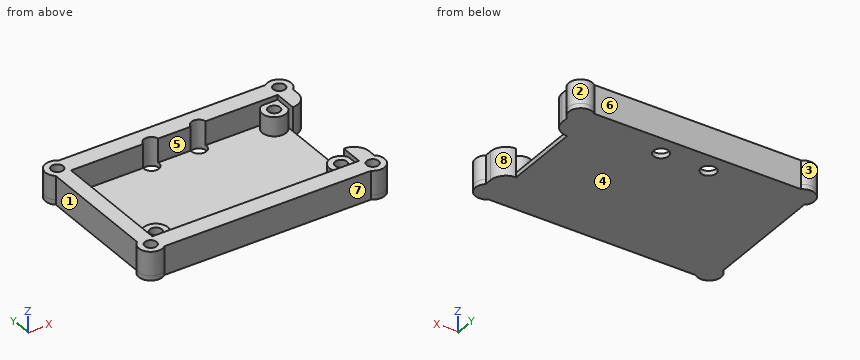
from build123d import *

# Parameters (mm, degrees)
SKETCH_R                   = 2.5
SKETCH_W                   = 87
SKETCH_H                   = 51
PAD_DEPTH                  = 10
POCKET_DEPTH               = 10.001
PAD001_DEPTH               = 2
SKETCH003_R                = 2.5
PAD002_DEPTH               = 8
SKETCH003_MIRRORED001_2_R  = 2.5
PAD002_MIRRORED001_2_DEPTH = 8
SKETCH004_R                = 3.2
POCKET001_DEPTH            = 12.001
POCKET004_DEPTH            = 8


with BuildPart() as part:
    # Sketch → Pad (new body)
    with BuildSketch(Plane.XY):
        with BuildLine():
            Line((-43.499999, 33.160444), (43.499999, 33.160444))
            ThreePointArc((49.927876, 25.500001), (50.544139, 32.544145), (43.499999, 33.160444))
            Line((49.927876, 25.500001), (49.927876, -25.500001))
            ThreePointArc((43.499999, -33.160444), (50.544159, -32.544162), (49.927876, -25.500001))
            Line((43.499999, -33.160444), (-43.499999, -33.160444))
            ThreePointArc((-49.927876, -25.500001), (-50.544159, -32.544162), (-43.499999, -33.160444))
            Line((-49.927876, -25.500001), (-49.927876, 25.500001))
            ThreePointArc((-43.499999, 33.160444), (-50.544159, 32.544162), (-49.927876, 25.500001))
        make_face()
        with Locations((-46.713937, 29.330223)):
            Circle(SKETCH_R, mode=Mode.SUBTRACT)
        with Locations((46.713917, 29.330206)):
            Circle(SKETCH_R, mode=Mode.SUBTRACT)
        with Locations((46.713937, -29.330223)):
            Circle(SKETCH_R, mode=Mode.SUBTRACT)
        with Locations((-46.713937, -29.330223)):
            Circle(SKETCH_R, mode=Mode.SUBTRACT)
        Rectangle(SKETCH_W, SKETCH_H, mode=Mode.SUBTRACT)
    extrude(amount=PAD_DEPTH)

    # Sketch001 (on Face18 of Pad) → Pocket (cut, through all)
    with BuildSketch(Plane.XY.offset(10)):
        with BuildLine():
            ThreePointArc((43.5, 16), (48.045195, 17.882681), (49.927876, 22.427876))
            Line((49.927876, 22.427876), (49.927876, -22.427876))
            ThreePointArc((49.927876, -22.427876), (48.045195, -17.882681), (43.5, -16))
            Line((43.5, 16), (43.5, -16))
        make_face()
    extrude(amount=-POCKET_DEPTH, mode=Mode.SUBTRACT)

    # Sketch002 (on Face4 of Pocket) → Pad001 (join)
    with BuildSketch(Plane(origin=(0, 0, 0), x_dir=(1, 0, 0), z_dir=(0, 0, -1))):
        with BuildLine():
            ThreePointArc((-43.499999, 33.160444), (-50.544168, 32.544169), (-49.927876, 25.500001))
            Line((-49.927876, 0), (-49.927876, 25.500001))
            Line((43.5, 0), (-49.927876, 0))
            Line((43.5, 16), (43.5, 0))
            ThreePointArc((43.5, 16), (48.045195, 17.882681), (49.927876, 22.427876))
            Line((49.927876, 25.500001), (49.927876, 22.427876))
            ThreePointArc((49.927876, 25.500001), (50.544166, 32.544167), (43.499999, 33.160444))
            Line((-43.499999, 33.160444), (43.499999, 33.160444))
        make_face()
    pad001 = extrude(amount=PAD001_DEPTH)

    # Mirrored: Pad001 across XZ
    add(pad001.mirror(Plane.XZ))

    # Sketch003 (on Face31 of Mirrored) → Pad002 (join)
    with BuildSketch(Plane.XY):
        with BuildLine():
            Line((36.820551, 25.5), (43.5, 25.5))
            Line((43.5, 25.5), (43.5, 18.820551))
            ThreePointArc((36.820551, 25.5), (35.464466, 17.464466), (43.5, 18.820551))
        make_face()
        with Locations((39, 21)):
            Circle(SKETCH003_R, mode=Mode.SUBTRACT)
    pad002 = extrude(amount=PAD002_DEPTH)

    # Sketch003 Mirrored001 2 → Pad002 Mirrored001 2 (add)
    with BuildSketch(Plane(origin=(0, 0, 0), x_dir=(-1, 0, 0), z_dir=(0, 0, -1))):
        with BuildLine():
            Line((36.820551, 25.5), (43.5, 25.5))
            Line((43.5, 25.5), (43.5, 18.820551))
            ThreePointArc((36.820551, 25.5), (35.464466, 17.464466), (43.5, 18.820551))
        make_face()
        with Locations((39, 21)):
            Circle(SKETCH003_MIRRORED001_2_R, mode=Mode.SUBTRACT)
    pad002_mirrored001_2 = extrude(amount=-PAD002_MIRRORED001_2_DEPTH)

    # Mirrored002: Pad002, Pad002 Mirrored001 2 across Sketch003 H_Axis
    add(pad002.mirror(Plane.ZX))
    add(pad002_mirrored001_2.mirror(Plane.ZX))

    # Sketch004 (on Face8 of MultiTransform) → Pocket001 (cut, through all)
    with BuildSketch(Plane(origin=(0, 0, -2), x_dir=(1, 0, 0), z_dir=(0, 0, -1))):
        with Locations((-10, -25)):
            Circle(SKETCH004_R)
        with Locations((10, -25)):
            Circle(SKETCH004_R)
    extrude(amount=-POCKET001_DEPTH, mode=Mode.SUBTRACT)

    # Sketch011 (on Face36 of Pocket001) → Pocket004 (cut)
    with BuildSketch(Plane.XY.offset(8)):
        with BuildLine():
            Line((-36.820551, 25.5), (-43.5, 25.5))
            Line((-43.5, 25.5), (-43.5, 18.820551))
            ThreePointArc((-43.5, 18.820551), (-35.464466, 17.464466), (-36.820551, 25.5))
        make_face()
    extrude(amount=-POCKET004_DEPTH, mode=Mode.SUBTRACT)


with BuildPart() as part_1:
    # Body placement: moved
    add(part.part.moved(Location((0, 0, -8))))


solid = part_1.part
The model under review builds one solid part; all positions refer to its coordinate system, in mm. Face numbers are marked on the shaded views. A direction names the side the tool comes from. Give positions to 0.01 mm unless a question says otherwise; leave off trailing zeros. Write each loop counter-clockwise with the first axis right and the second up, starting at its lowest first coordinate (ties: lowest second). Pieces come first, ordered by that corner, then holes. Notation, with made-up numbers: M -5,-1.5 L 32,-1.5 A26 cw 32,25.5 Z; hole C 66,32.5 d7. An arc over 180 degrees is marked long. One line per question, with ' | ' between items. Start each with the question number.
Item 1: Wall thickness on line 1 (Y direction, x = 39, z = -2); line 2 (Y direction, x = 3.5, z = -2.5); line 3 (X direction, y = -21, z = -3): over which ranges is each line inside the solid? List them lowest first. Write a range as from..to.
Item 2: We need section A-A on z = -9. Write out the cut boundary in (x, y).
Item 3: We need section B-B on x = -10. Write out the cut boundary in (y, z).
Item 4: We need section D-D on z = -1.25. Give the number of separate pieces and of enclosed holes in the cut face, plus the area to 3 significant figures.
Item 5: Draft analysis for pull direction X (two halves, no side actions). For the marked faces 1, 2, 3 and 4, state which applies: released by +X, released by -X, zero draft, split by the parting line, or undercut.
Item 6: For the marked faces 5, 6, 7 and 8, list the 3-axis set-ups (+Z, -Z, +X, -X, +Y, -Y) from which the entire face can be reached by the end or side of a thin tool; tool diameter is ignored.
Item 7: We need section C-C on x = -39. Write out the cut boundary in (y, z), plus the area to 3 significant figures.
Item 8: For pin 1 (2.5 mm diameter, centred on x = 46.5, y = 30, fed in from +Z); pin 2 (1 mm diameter, centred on y = -17.5, z = -1, fed in from +X); pin 3 (1.5 mm diameter, centred on x = -18, z = -3.5, fed in from +Y), all flat-tipped, find the tip position at first contact; note any pin that passes through.
Results found:
1) line 1: y = -33.16..-23.5, -18.5..-16, 16..18.5, 23.5..33.16 | line 2: y = -33.16..-25.5, 25.5..33.16 | line 3: x = -49.93..-41.5, -36.5..-34, 34..36.5, 41.5..49.77
2) outline: M -49.93,-25.5 A5 ccw -43.5,-33.16 L 43.5,-33.16 A5 ccw 49.93,-25.5 L 49.93,-22.43 A6.43 ccw 43.5,-16 L 43.5,16 A6.43 ccw 49.93,22.43 L 49.93,25.5 A5 ccw 43.5,33.16 L -43.5,33.16 A5 ccw -49.93,25.5 Z; hole C -10,25 d6.4; hole C 10,25 d6.4
3) outline: M -33.16,-10 L 21.8,-10 L 21.8,-8 L -25.5,-8 L -25.5,2 L -33.16,2 Z; M 28.2,-10 L 33.16,-10 L 33.16,2 L 28.2,2 Z
4) separate pieces: 1 | enclosed holes: 7 | area: 2,090 mm2
5) face 1: released by -X | face 2: undercut | face 3: undercut | face 4: zero draft
6) face 5: +Z | face 6: +Z, -Z, +Y | face 7: +Z, -Z, -Y | face 8: +Z, -Z, +X
7) outline: M -33.16,-10 L 33.16,-10 L 33.16,2 L 25.5,2 L 25.5,-8 L -16,-8 L -16,0 L -18.5,0 L -18.5,-8 L -23.5,-8 L -23.5,0 L -25.5,0 L -25.5,2 L -33.16,2 Z | area: 322 mm2
8) pin 1: stops at z = -8 | pin 2: stops at x = 48.16 | pin 3: stops at y = 33.16
